Job drawing, mm, ordinate dimensions from the low corner. One solid piece. A direction names the side the tool comes from. Give positions to 0.01 mm unless a question says otherwise; leave off trailing zeros. Order: outer loops, then holes, each group sorted by start corner. A loop starts at its lowest first (then second) coordinate and runs counter-clockwise, first axis right, second up. Notation, with made-up numbers: M 81,30 L 138,30 A29 ccw 138,66 Z; hole C -30.5,78 d7. An arc over 180 degrees is marked long. Use CSV: the item, a comma, the result in double quotes. Start each with the question number.
Item 1: Pin check, flat tips, straight feed: P1, Ø4, axis at x = 3.5, z = 8, coming from the -Y side; P2, Ø2, axis at x = 3, z = 13, coming from the +Y side; P3, Ø4, axis at x = 3, z = 9.5, coming from the -Y side. Stop position of each tip, or through.
Item 2: Which spindle directions (+Z, -Z, +X, -X, +Y, -Y) get a long thin tool onto all of the face, cutting with end or side? Do the marked faces 1 and 2. Say none if no direction does.
Item 3: Two-plate mould, pull along Y, no slides. Class the marked faces 3, 4 and 5: pulls with the +Y half, pulls with the -Y half, needs draft (parallel to the pull), parting line crosses it, or undercut.
Item 4: Band-saw the part on B-B on z = 6. Write the cut outline in (x, y), plus the area to 3 significant figures.
Item 5: Wall check: line 1 along Y through (x, z) = (6, 8.75); line 2 along Z through (x, y) = (3.5, 15); line 3 along Y through (x, z) = (6, 15). Give the ranges that are in metal, low to high.
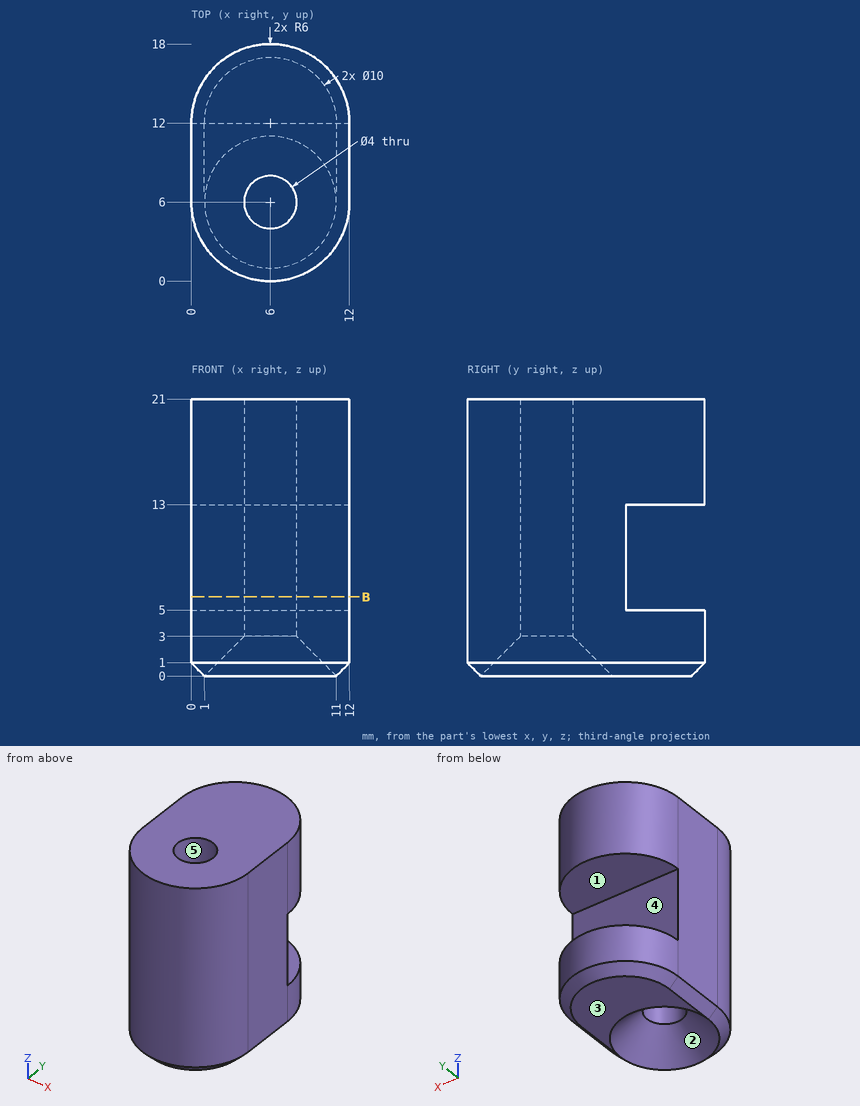
Model answer:
1,P1,"stops at y = 0.02"
1,P2,"stops at y = 17.66"
1,P3,"stops at y = 0.08"
2,face 1,"+X, -X, +Y"
2,face 2,"-Z"
3,face 3,"needs draft"
3,face 4,"pulls with the +Y half"
3,face 5,"undercut"
4,outline,"M 0,6 A6 ccw 12,6 L 12,12 L 0,12 Z; hole C 6,6 d4"
4,area,"116 mm^2"
5,line 1,"y = 0 to 4, 8 to 12"
5,line 2,"z = 0 to 5, 13 to 21"
5,line 3,"y = 0 to 4, 8 to 18"
